from build123d import *

# Parameters (mm, degrees)
SKETCH2_R               = 4.1
SKETCH2_R_2             = 2.6
BOSS_EXTRUDE1_DEPTH     = 7
SKETCH3_R               = 8
SKETCH3_R_2             = 2.6
BOSS_EXTRUDE2_DEPTH     = 7.5
SKETCH4_R               = 1.31
CUT_EXTRUDE1_DEPTH      = 9
CUT_EXTRUDE2_DEPTH      = 5
CUT_EXTRUDE2_DEPTH_BACK = 2
SKETCH5_R               = 1.31


with BuildPart() as part:
    # Sketch2 → Boss-Extrude1 (new body)
    # profile 1 of 2: a face of its own
    with BuildSketch(Plane.XY):
        with BuildLine():
            ThreePointArc((-8.388352144, 2.232508627), (-7.643352144, 2.753972912), (-8.388352144, 3.275437196))
            Line((-8.388352144, 3.275437196), (-8.388352144, 4.232508627))
            ThreePointArc((-8.388352144, 4.232508627), (-7.805907881, 4.361528648), (-7.67688786, 4.943972912))
            Line((-7.67688786, 4.943972912), (-6.719816429, 4.943972912))
            ThreePointArc((-6.719816429, 4.943972912), (-6.198352144, 4.198972912), (-5.67688786, 4.943972912))
            Line((-5.67688786, 4.943972912), (-4.719816429, 4.943972912))
            ThreePointArc((-4.719816429, 4.943972912), (-4.198352144, 4.198972912), (-3.67688786, 4.943972912))
            Line((-3.67688786, 4.943972912), (-2.719816429, 4.943972912))
            ThreePointArc((-2.719816429, 4.943972912), (-2.198352144, 4.198972912), (-1.67688786, 4.943972912))
            Line((-1.67688786, 4.943972912), (-0.719816429, 4.943972912))
            ThreePointArc((-0.719816429, 4.943972912), (-0.198352144, 4.198972912), (0.32311214, 4.943972912))
            Line((0.32311214, 4.943972912), (1.280183571, 4.943972912))
            ThreePointArc((1.280183571, 4.943972912), (1.409203592, 4.361528648), (1.991647856, 4.232508627))
            Line((1.991647856, 4.232508627), (1.991647856, 3.275437196))
            ThreePointArc((1.991647856, 3.275437196), (1.246647856, 2.753972912), (1.991647856, 2.232508627))
            Line((1.991647856, 2.232508627), (1.991647856, 1.275437196))
            ThreePointArc((1.991647856, 1.275437196), (1.246647856, 0.753972912), (1.991647856, 0.232508627))
            Line((1.991647856, 0.232508627), (1.991647856, -0.724562804))
            ThreePointArc((1.991647856, -0.724562804), (1.246647856, -1.246027088), (1.991647856, -1.767491373))
            Line((1.991647856, -1.767491373), (1.991647856, -2.724562804))
            ThreePointArc((1.991647856, -2.724562804), (1.246647856, -3.246027088), (1.991647856, -3.767491373))
            Line((1.991647856, -3.767491373), (1.991647856, -4.724562804))
            ThreePointArc((1.991647856, -4.724562804), (1.409203592, -4.853582824), (1.280183571, -5.436027088))
            Line((1.280183571, -5.436027088), (0.32311214, -5.436027088))
            ThreePointArc((0.32311214, -5.436027088), (-0.198352144, -4.691027088), (-0.719816429, -5.436027088))
            Line((-0.719816429, -5.436027088), (-1.67688786, -5.436027088))
            ThreePointArc((-1.67688786, -5.436027088), (-2.198352144, -4.691027088), (-2.719816429, -5.436027088))
            Line((-2.719816429, -5.436027088), (-3.67688786, -5.436027088))
            ThreePointArc((-3.67688786, -5.436027088), (-4.198352144, -4.691027088), (-4.719816429, -5.436027088))
            Line((-4.719816429, -5.436027088), (-5.67688786, -5.436027088))
            ThreePointArc((-5.67688786, -5.436027088), (-6.198352144, -4.691027088), (-6.719816429, -5.436027088))
            Line((-6.719816429, -5.436027088), (-7.67688786, -5.436027088))
            ThreePointArc((-7.67688786, -5.436027088), (-7.805907881, -4.853582824), (-8.388352144, -4.724562804))
            Line((-8.388352144, -4.724562804), (-8.388352144, -3.767491373))
            ThreePointArc((-8.388352144, -3.767491373), (-7.643352144, -3.246027088), (-8.388352144, -2.724562804))
            Line((-8.388352144, -2.724562804), (-8.388352144, -1.767491373))
            ThreePointArc((-8.388352144, -1.767491373), (-7.643352144, -1.246027088), (-8.388352144, -0.724562804))
            Line((-8.388352144, -0.724562804), (-8.388352144, 0.232508627))
            ThreePointArc((-8.388352144, 0.232508627), (-7.643352144, 0.753972912), (-8.388352144, 1.275437196))
            Line((-8.388352144, 1.275437196), (-8.388352144, 2.232508627))
        make_face()
        with Locations((-3.198352144, -0.246027088)):
            Circle(SKETCH2_R, mode=Mode.SUBTRACT)
    # profile 2 of 2: a face of its own
    with BuildSketch(Plane.XY):
        with Locations((-3.198352144, -0.246027088)):
            Circle(SKETCH2_R)
        with Locations((-3.198352144, -0.246027088)):
            Circle(SKETCH2_R_2, mode=Mode.SUBTRACT)
    extrude(amount=BOSS_EXTRUDE1_DEPTH)

    # Sketch3 → Boss-Extrude2 (add)
    with BuildSketch(Plane.XY.offset(7)):
        with Locations((-3.198352144, -0.246027088)):
            Circle(SKETCH3_R)
        with Locations((-3.198352144, -0.246027088)):
            Circle(SKETCH3_R_2, mode=Mode.SUBTRACT)
    extrude(amount=BOSS_EXTRUDE2_DEPTH)

    # Sketch4 → Cut-Extrude1 (cut)
    with BuildSketch(Plane(origin=(0, 0, 0), x_dir=(1, 0, 0), z_dir=(0, 1, 0))):
        with Locations(Location((-3.198352144, -10.75, 0), (0, 0, 270))):
            Circle(SKETCH4_R)
    extrude(amount=-CUT_EXTRUDE1_DEPTH, mode=Mode.SUBTRACT)

    # Sketch5 → Cut-Extrude2 (cut, two sides: drawn at the far end of the back side and taken through both)
    with BuildSketch(Plane(origin=(0, 0, 0), x_dir=(0, 0, -1), z_dir=(1, 0, 0)).offset(-CUT_EXTRUDE2_DEPTH_BACK)):
        with Locations((-10.75, -0.246027088)):
            Circle(SKETCH5_R)
    extrude(amount=CUT_EXTRUDE2_DEPTH + CUT_EXTRUDE2_DEPTH_BACK, mode=Mode.SUBTRACT)


solid = part.part
Verification items for the finished model (mm, model axes). A direction names the side the tool comes from. Give positions to 0.01 mm unless a question says otherwise; leave off trailing zeros. Write each loop counter-clockwise with the first axis right and the second up, starting at its lowest first coordinate (ties: lowest second). Pieces come first, ordered by that corner, then holes. Notation, with made-up numbers: (48, -32) - (66, -32) arc R22 cw to (66, -16) - close; hole circle Ø9 at (31, 17). An arc over 180 degrees is marked (long way). Answer as CSV lines item,"result". Start each with the question number.
1. Set-up check for faces 1 (the face through (1.88, -0.19, 12.06)), 2 (the face through (1.992, 2, 3)), 3 (the face through (-1, 4.944, 3)), 4 (the face through (-8.388, -4, 3)), 5 (the face through (1.247, -3.231, 3.451)): record each of +Z, -Z, +X, -X, +Y, -Y from which the full face is reachable in a straight line by a thin tool's end or side.
2. Draft check along X on faces 6 (the face through (-5, -5.436, 3)), 7 (the face through (-3.14, -5.33, 9.44)), 8 (the face through (1.992, 4, 3)), 9 (the face through (-7.644, 0.739, 3.451)). Enter one of: pulls with the +X half, pulls with the -X half, needs draft (parallel to the pull), parting line crosses it, or undercut.
3. Sectioned sample at A-A (y = -3.5). Record the boundary of the cut face in (x, z).
4. Thickness scan on line 1 (Y direction, x = -3.5, z = 1.75); line 2 (Y direction, x = -2.5, z = 9.25); line 3 (Z direction, x = -4, y = 6.5). Record the ranges inside material, lowest first.
5. Sectioned sample at C-C (x = -7). Record the boundary of the cut face in (y, z).
6. Depth check by flat-ended pin: pin 1 (1.1 mm diameter, centred on x = -7, z = 3, fed in from -Y); pin 2 (0.8 mm diameter, centred on x = -5, z = 2, fed in from +Y); pin 3 (1.4 mm diameter, centred on x = 1.8, y = 0.75, fed in from -Z); pin 4 (0.8 mm diameter, centred on y = -2.5, z = 4, fed in from +X). Enter the tip coordinate at first touch or a pass-through.
7. Sectioned sample at B-B (z = 10.75). Record the boundary of the cut face in (x, y).
8. Sectioned sample at D-D (y = 4.5). Record the boundary of the cut face in (x, z).
Derived:
1,face 1,"+X"
1,face 2,"-Z, +X, +Y, -Y"
1,face 3,"-Z, +X, -X, +Y"
1,face 4,"-Z, -X, +Y, -Y"
1,face 5,"-Z"
2,face 6,"needs draft"
2,face 7,"undercut"
2,face 8,"pulls with the +X half"
2,face 9,"undercut"
3,outline,"(-10.51, 7) - (-7.7, 7) - (-7.7, 0) - (1.31, 0) - (1.31, 7) - (4.11, 7) - (4.11, 14.5) - (-10.51, 14.5) - close; hole circle Ø2.62 at (-3.2, 10.75)"
4,line 1,"-5.44 to -2.83, 2.34 to 4.94"
4,line 2,"-8.22 to -2.75, 2.26 to 7.72"
4,line 3,"7 to 14.5"
5,outline,"(-7.29, 7) - (-5.44, 7) - (-5.44, 0) - (4.94, 0) - (4.94, 7) - (6.79, 7) - (6.79, 14.5) - (-7.29, 14.5) - close"
6,pin 1,"y = -5.44"
6,pin 2,"y = 4.94"
6,pin 3,"z = 0"
6,pin 4,"x = 1.99"
7,outline,"(-4.51, -8.14) - (-4.51, -2.49) arc R2.6 cw (long way) to (-0.95, 1.06) - (4.69, 1.06) arc R8 ccw (long way) to start; (-1.89, -8.14) arc R8 ccw to (4.69, -1.56) - (-0.95, -1.56) arc R2.6 cw to (-1.89, -2.49) - close"
8,outline,"(-9.64, 7) - (-7.7, 7) - (-7.7, 0) - (-6.69, 0) - (-6.69, 7) - (-5.7, 7) - (-5.7, 0) - (-4.69, 0) - (-4.69, 7) - (-3.7, 7) - (-3.7, 0) - (-2.69, 0) - (-2.69, 7) - (-1.7, 7) - (-1.7, 0) - (-0.69, 0) - (-0.69, 7) - (0.3, 7) - (0.3, 0) - (1.31, 0) - (1.31, 7) - (3.24, 7) - (3.24, 14.5) - (-9.64, 14.5) - close"
